Work out the finished part from the listing and answer in its coordinate system (mm). Coordinates: 2 decimals unless noted, no trailing zeros. Write each loop counter-clockwise with the first axis right and the second up, starting at its lowest first coordinate (ties: lowest second). Pieces come first, ordered by that corner, then holes. Notation, with made-up numbers: (-2, 62.5) - (44, 62.5) arc R19 cw to (44, 77.5) - close; hole circle Ø1 at (57.25, -26.5). An arc over 180 degrees is marked (long way). Answer as a JSON object with one key per item and string values. Group by question number.
from build123d import *

# Parameters (mm, degrees)
SKETCH1_W              = 40
SKETCH1_H              = 200
BOSS_EXTRUDE1_DEPTH    = 10
SKETCH2_W              = 15
SKETCH2_H              = 150
BOSS_EXTRUDE2_DEPTH    = 8
FILLET1_R              = 10
CUT_EXTRUDE1_DEPTH     = 205.753510348
FILLET2_R              = 4
SPLIT1_SURFACE_1_BACK  = 205.754
SPLIT1_SURFACE_1_DEPTH = 411.508


with BuildPart() as part:
    # Sketch1 → Boss-Extrude1 (new body)
    with BuildSketch(Plane(origin=(0, 0, 0), x_dir=(1, 0, 0), z_dir=(0, 1, 0))):
        with Locations((20, 100)):
            Rectangle(SKETCH1_W, SKETCH1_H)
    extrude(amount=BOSS_EXTRUDE1_DEPTH)

    # Sketch2 → Boss-Extrude2 (add)
    with BuildSketch(Plane(origin=(0, 10, 0), x_dir=(1, 0, 0), z_dir=(0, 1, 0))):
        with Locations((20, 100)):
            Rectangle(SKETCH2_W, SKETCH2_H)
    extrude(amount=BOSS_EXTRUDE2_DEPTH)

    # Fillet1
    fillet1_edges = [part.edges().sort_by_distance(p)[0] for p in [
        (27.5, 14, -25),
        (27.5, 14, -175),
    ]]
    fillet(fillet1_edges, radius=FILLET1_R)

    # Sketch3 → Cut-Extrude1 (cut, through all)
    with BuildSketch(Plane.XY):
        Polygon((27.5, 18), (12.5, 18), (12.5, 10), align=None)
    extrude(amount=-CUT_EXTRUDE1_DEPTH, mode=Mode.SUBTRACT)

    # Fillet2
    fillet2_edges = [part.edges().sort_by_distance(p)[0] for p in [
        (12.5, 10, -100),
    ]]
    fillet(fillet2_edges, radius=FILLET2_R)

    # Split1: cut with a surface, the side it looks to stays
    # Split1 surface: a surface, the sketch's curves swept straight by 411.508 mm
    with BuildLine(Plane.XY.offset(-SPLIT1_SURFACE_1_BACK), mode=Mode.PRIVATE) as split1_surface_1_path:
        Line((0, 10), (40, 10))
    split1_surface_1 = Shell.extrude(split1_surface_1_path.wire(), (0 * SPLIT1_SURFACE_1_DEPTH, 0 * SPLIT1_SURFACE_1_DEPTH, 1 * SPLIT1_SURFACE_1_DEPTH))
    split(bisect_by=split1_surface_1, keep=Keep.TOP)


solid = part.part
Q1. Section B-B on x = 19.75 is taken. Determine the outline of the cut face in (y, z).
Q2. Consider L1, parallel to X at y = 16, z = -70.5; L2, parallel to Y at x = 13.5, z = -54; L3, parallel to X at y = 16.25, z = -137. Determine where each line is inside the solid, lowest interval first. Write a range as from..to.
Q3. A flat-ended cylindrical pin translates along its axis: pin 1 Ø1.5 at (x, z) = (15.5, -130.5) entering from +Y. Find the tip coordinate at first contact, or state that the pin passes through.
Q4. Section A-A on z = -75.5 is taken. Determine the outline of the cut face in (x, y), plus the area to 3 significant figures.
Numbers:
{
 "1": {"outline": "(10, -174.74) - (13.87, -174.74) - (13.87, -25.26) - (10, -25.26) - close"},
 "2": {"L1": "x = 23.75..27.5", "L2": "y = 10..10.53", "L3": "x = 24.22..27.5"},
 "3": {"pin 1": "stops at y = 12"},
 "4": {"outline": "(11.5, 10) - (27.5, 10) - (27.5, 18) - (13.38, 10.47) arc R4 cw to start", "area": "60.1 mm²"}
}
